from build123d import *

# Parameters (mm, degrees)
SHELL1_START        = -169
SHELL1_DEPTH        = 196.698454184
BOSS_EXTRUDE1_REACH = 223.544
SKETCH5_W           = 20
SKETCH5_H           = 3
SKETCH6_W           = 20
SKETCH6_H           = 3
BOSS_EXTRUDE2_DEPTH = 79.88011004
CUT_EXTRUDE1_REACH  = 187.712
SKETCH7_W           = 20
SKETCH7_H           = 20
BOSS_EXTRUDE3_DEPTH = 2
FILLET1_R           = 2
CUT_EXTRUDE2_REACH  = 187.712
SKETCH9_R           = 2.75


with BuildPart() as part:
    # Loft1: read off the stored shape, not the designer's step
    # Loft1: loft between two sections, ruled curve by curve
    loft1_from = [
        Edge.make_line((40.035, 150, -9.025), (-80.035, 150, -9.025)),
        Edge.make_line((-80.035, 150, -9.025), (-80.035, 150, -30.975)),
        Edge.make_line((40.035, 150, -30.975), (40.035, 150, -9.025)),
        Edge.make_line((-80.035, 150, -30.975), (40.035, 150, -30.975)),
    ]
    loft1_to = [
        Edge.make_line((80.035, 0, 30.975), (-80.035, 0, 30.975)),
        Edge.make_line((-80.035, 0, 30.975), (-80.035, 0, -30.975)),
        Edge.make_line((80.035, 0, -30.975), (80.035, 0, 30.975)),
        Edge.make_line((-80.035, 0, -30.975), (80.035, 0, -30.975)),
    ]
    loft1 = Solid(Shell([*[Face.make_surface_from_curves(loft1_from[k], loft1_to[k]) for k in range(4)], Face(Wire(loft1_from)), Face(Wire(loft1_to))]))
    add(loft1)

    # Shell1: read off the stored shape, not the designer's step
    # Shell1 outline → Shell1 (cut)
    with BuildSketch(Plane(origin=(0, 0, 0), x_dir=(0.9683714115263207, 0.24108831822232024, -0.06429021819261868), z_dir=(0.2495131446207219, -0.935674292327708, 0.2495131446207219)).offset(SHELL1_START)):
        Polygon((73.640867828, 27.929127254), (-81, 27.929127254), (-81, -31), (77.561825655, -31), (77.490573168, -29.929127254), align=None)
    extrude(amount=SHELL1_DEPTH, mode=Mode.SUBTRACT)

    # Boss-Extrude1: up to this plane
    boss_extrude1_end = Plane(origin=(74.721473029, 19.925726141, 0), z_dir=(0.9662349396012464, 0.2576626505603324, 0))
    # Sketch5 → Boss-Extrude1 (add, up to the surface)
    with BuildSketch(Plane.ZY.offset(80.035), mode=Mode.PRIVATE) as boss_extrude1_sk1:
        with Locations((38.90511004, 1.5)):
            Rectangle(SKETCH5_W, SKETCH5_H)
    boss_extrude1_tool1 = split(extrude(boss_extrude1_sk1.sketch, amount=-BOSS_EXTRUDE1_REACH, mode=Mode.PRIVATE), bisect_by=boss_extrude1_end, keep=Keep.BOTH, mode=Mode.PRIVATE)
    add(boss_extrude1_tool1.solids().sort_by_distance((-80.035, 1.5, 38.90511))[0])

    # Sketch6 → Boss-Extrude2 (add)
    with BuildSketch(Plane(origin=(0, 0, -30.975), x_dir=(-1, 0, 0), z_dir=(0, 0, -1))):
        with Locations((-87.96511004, 1.5)):
            Rectangle(SKETCH6_W, SKETCH6_H)
    extrude(amount=-BOSS_EXTRUDE2_DEPTH)

    # Sketch7 → Cut-Extrude1 (cut, up to next)
    with BuildSketch(Plane(origin=(0, 0, 0), x_dir=(-1, 0, 0), z_dir=(0, -1, 0)), mode=Mode.PRIVATE) as cut_extrude1_sk1:
        with Locations((-87.96511004, -38.90511004)):
            Rectangle(SKETCH7_W, SKETCH7_H)
    cut_extrude1_tool1 = extrude(cut_extrude1_sk1.sketch, amount=-CUT_EXTRUDE1_REACH, mode=Mode.PRIVATE) & part.part
    add(cut_extrude1_tool1.solids().sort_by_distance((87.96511, 0, 38.90511))[0], mode=Mode.SUBTRACT)

    # Sketch8 → Boss-Extrude3 (add)
    with BuildSketch(Plane.ZY.offset(80.035)):
        Polygon((28.90511004, 0), (-30.975, 0), (-30.975, 150), (-11.09488996, 150), (-9.025, 150), (30.175, 3), (48.90511004, 3), (48.90511004, 0), align=None)
    extrude(amount=BOSS_EXTRUDE3_DEPTH)

    # Fillet1
    # the kernel refuses this fillet: 2 mm, written as the material it adds along each edge
    with BuildSketch(Plane(origin=(36.797794865, 154.377431907, -12.262205135), x_dir=(0.06429021819457766, -0.24108831822179794, -0.9683714115263207), z_dir=(0.24951314462072197, -0.9356742923277082, 0.24951314462072197))) as fillet1_piece_1_section:
        with BuildLine():
            CenterArc((FILLET1_R * 0.935674292326, -FILLET1_R), FILLET1_R, 90, 86.193330917)
            Line((-FILLET1_R * 0.0621194550941, -FILLET1_R * 0.933609958504), (0, 0))
            Line((0, 0), (FILLET1_R * 0.935674292326, 0))
        make_face()
    fillet1_piece_1 = extrude(amount=172.943798365, mode=Mode.PRIVATE)
    fillet1_piece_1 = split(fillet1_piece_1, bisect_by=Plane(origin=(36.797794865, 150, -12.262205135), z_dir=(0, -1, 0)), keep=Keep.TOP, mode=Mode.PRIVATE)
    fillet1_piece_1 = split(fillet1_piece_1, bisect_by=Plane(origin=(36.797794865, 0, -12.262205135), z_dir=(0, 1, 0)), keep=Keep.TOP, mode=Mode.PRIVATE)
    add(fillet1_piece_1)
    with BuildSketch(Plane(origin=(-80.035, 154.831174698, -12.383203212), x_dir=(1, 0, 0), z_dir=(0, -0.9662349396012464, 0.2576626505603321))) as fillet1_piece_2_section:
        with BuildLine():
            CenterArc((FILLET1_R, -FILLET1_R), FILLET1_R, 90, 90)
            Line((0, -FILLET1_R), (0, 0))
            Line((0, 0), (FILLET1_R, 0))
        make_face()
    fillet1_piece_2 = extrude(amount=165.241746963, mode=Mode.PRIVATE)
    fillet1_piece_2 = split(fillet1_piece_2, bisect_by=Plane(origin=(-80.035, 150, -12.383203212), z_dir=(0, -1, 0)), keep=Keep.TOP, mode=Mode.PRIVATE)
    fillet1_piece_2 = split(fillet1_piece_2, bisect_by=Plane(origin=(-80.035, 0, -12.383203212), z_dir=(0, 1, 0)), keep=Keep.TOP, mode=Mode.PRIVATE)
    add(fillet1_piece_2)

    # Sketch9 → Cut-Extrude2 (cut, up to next)
    with BuildSketch(Plane.XZ, mode=Mode.PRIVATE) as cut_extrude2_sk1:
        with Locations(Location((87.96511004, -15.975, 0), (0, 0, 270))):
            Circle(SKETCH9_R)
    cut_extrude2_tool1 = extrude(cut_extrude2_sk1.sketch, amount=-CUT_EXTRUDE2_REACH, mode=Mode.PRIVATE) & part.part
    # Sketch9 → Cut-Extrude2 (cut, up to next)
    with BuildSketch(Plane.XZ, mode=Mode.PRIVATE) as cut_extrude2_sk2:
        with Locations(Location((87.96511004, 13.90511004, 0), (0, 0, 270))):
            Circle(SKETCH9_R)
    cut_extrude2_tool2 = extrude(cut_extrude2_sk2.sketch, amount=-CUT_EXTRUDE2_REACH, mode=Mode.PRIVATE) & part.part
    # Sketch9 → Cut-Extrude2 (cut, up to next)
    with BuildSketch(Plane.XZ, mode=Mode.PRIVATE) as cut_extrude2_sk3:
        with Locations(Location((62.96511004, 38.90511004, 0), (0, 0, 270))):
            Circle(SKETCH9_R)
    cut_extrude2_tool3 = extrude(cut_extrude2_sk3.sketch, amount=-CUT_EXTRUDE2_REACH, mode=Mode.PRIVATE) & part.part
    # Sketch9 → Cut-Extrude2 (cut, up to next)
    with BuildSketch(Plane.XZ, mode=Mode.PRIVATE) as cut_extrude2_sk4:
        with Locations(Location((-67.035, 38.90511004, 0), (0, 0, 270))):
            Circle(SKETCH9_R)
    cut_extrude2_tool4 = extrude(cut_extrude2_sk4.sketch, amount=-CUT_EXTRUDE2_REACH, mode=Mode.PRIVATE) & part.part
    add(cut_extrude2_tool1.solids().sort_by_distance((87.96511, 0, -15.975))[0], mode=Mode.SUBTRACT)
    add(cut_extrude2_tool2.solids().sort_by_distance((87.96511, 0, 13.90511))[0], mode=Mode.SUBTRACT)
    add(cut_extrude2_tool3.solids().sort_by_distance((62.96511, 0, 38.90511))[0], mode=Mode.SUBTRACT)
    add(cut_extrude2_tool4.solids().sort_by_distance((-67.035, 0, 38.90511))[0], mode=Mode.SUBTRACT)


solid = part.part
Design review of the part built by this model. Coordinates are the model's own, in mm. A direction names the side the tool comes from. Round coordinates to 2 decimals unless told otherwise and drop trailing zeros. One line per question, with ' | ' between items.
1. For faces 5 (the face through (-1, 3, 39)), 6 (the face through (89, 3, -1)), 7 (the face through (-79.434, 76.164, 8.004)), 8 (the face through (77.965, 2, 39)), list the 3-axis set-ups (+Z, -Z, +X, -X, +Y, -Y) from which the entire face can be reached by the end or side of a thin tool; tool diameter is ignored.
Results are:
face 5: +Z, +X, -X, +Y | face 6: +Z, -Z, +X, +Y | face 7: -Z, -Y | face 8: +Z, +X, +Y, -Y
2. Clearance check with flat-ended pins moving along their axes: P1, Ø8, axis at x = 31.5, y = 82.5, coming from the +Z side; P2, Ø1.5, axis at x = 3.5, y = 39, coming from the +Z side (3 decimals); P3, Ø6, axis at x = 92.5, y = 5, coming from the +Z side; P4, Ø9, axis at x = -67.04, z = 38.91, coming from the -Y side. State where each tip first meets the part, or that it passes through.
Results are:
P1: stops at z = 10.04 | P2: stops at z = 20.775 | P3: stops at z = 28.91 | P4: stops at y = 0
3. For L1, parallel to Y at x = -39, z = 31; L2, parallel to X at y = 144, z = -20 (3 decimals); L3, parallel to X at y = 80, z = -8.5 (3 decimals), list the stretches that pass through material, from the lowest coordinate up. Write a range as [from, to].
Results are:
L1: y = [0, 3] | L2: x = [-82.035, -80.035], [39.565, 41.635] | L3: x = [-82.035, -80.035], [56.632, 58.702]
4. Draft analysis for pull direction Z (two halves, no side actions). For faces 1 (the face through (-64.31, 1.48, 39.26)), 2 (the face through (57, 81, -30.975)), 3 (the face through (88.79, 1.48, -18.6)), 4 (the face through (63.115, 55.686, -10.818)), state which applies: released by +Z, released by -Z, zero draft, split by the parting line, or undercut.
Results are:
face 1: undercut | face 2: released by -Z | face 3: undercut | face 4: zero draft
